Work out the finished part from the listing and answer in its coordinate system (mm). Face numbers are marked on the shaded views. A direction names the side the tool comes from. Round coordinates to 2 decimals unless told otherwise and drop trailing zeros. Loops run counter-clockwise (first coordinate to the right, second up) from the corner with the lowest first, then second, coordinate; pieces in that order, holes last. Notation, with made-up numbers: (23.25, 8.5) -> (56.25, 8.5) arc R26 ccw to (56.25, 43.5) -> close; hole circle Ø6 at (5.25, -21.75). An arc over 180 degrees is marked (long way). Write item = value, one per line. Start each with the question number.
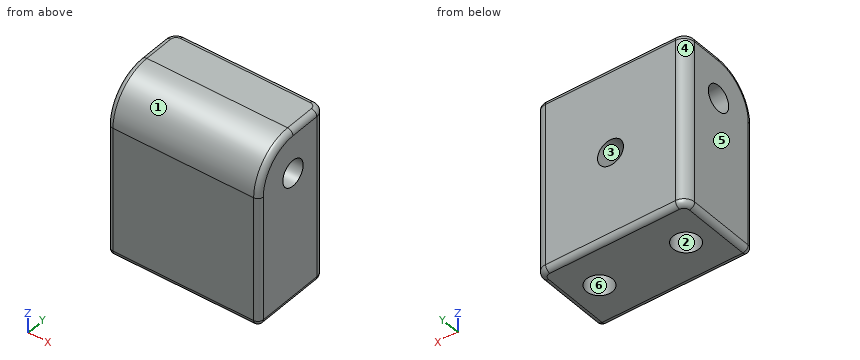
```python
from build123d import *

# Parameters (mm, degrees)
SKETCH1_R           = 1.905
BOSS_EXTRUDE1_DEPTH = 12.7
BOSS_EXTRUDE2_DEPTH = 12.7
CUT_EXTRUDE1_REACH  = 37.955
SKETCH3_R           = 1.905
SKETCH4_R           = 1.905
CUT_EXTRUDE2_DEPTH  = 10.8077
FILLET1_R           = 0.79375
FILLET2_R           = 6.35


with BuildPart() as part:
    # Sketch1 → Boss-Extrude1 (new body)
    with BuildSketch(Plane.XY):
        with BuildLine():
            Line((-11.1125, 0), (11.1125, 0))
            Line((11.1125, 0), (11.1125, 10.8077))
            ThreePointArc((11.1125, 10.8077), (10.647532015, 11.930232015), (9.525, 12.3952))
            Line((9.525, 12.3952), (-9.525, 12.3952))
            ThreePointArc((-9.525, 12.3952), (-10.647532015, 11.930232015), (-11.1125, 10.8077))
            Line((-11.1125, 10.8077), (-11.1125, 0))
        make_face()
        with Locations((-6.35, 6.35)):
            Circle(SKETCH1_R, mode=Mode.SUBTRACT)
        with Locations((6.35, 6.35)):
            Circle(SKETCH1_R, mode=Mode.SUBTRACT)
    extrude(amount=BOSS_EXTRUDE1_DEPTH)

    # Sketch2 → Boss-Extrude2 (add)
    with BuildSketch(Plane.XY.offset(12.7)):
        with BuildLine():
            Line((11.1125, 0), (11.1125, 10.8077))
            ThreePointArc((11.1125, 10.8077), (10.647532015, 11.930232015), (9.525, 12.3952))
            Line((9.525, 12.3952), (-9.525, 12.3952))
            ThreePointArc((-9.525, 12.3952), (-10.647532015, 11.930232015), (-11.1125, 10.8077))
            Line((-11.1125, 10.8077), (-11.1125, 0))
            Line((-11.1125, 0), (11.1125, 0))
        make_face()
    extrude(amount=BOSS_EXTRUDE2_DEPTH)

    # Sketch3 → Cut-Extrude1 (cut, up to next)
    with BuildSketch(Plane(origin=(11.1125, 0, 0), x_dir=(0, 0, -1), z_dir=(1, 0, 0)), mode=Mode.PRIVATE) as cut_extrude1_sk1:
        with Locations(Location((-19.05, 6.35, 0), (0, 0, 90))):
            Circle(SKETCH3_R)
    cut_extrude1_tool1 = extrude(cut_extrude1_sk1.sketch, amount=-CUT_EXTRUDE1_REACH, mode=Mode.PRIVATE) & part.part
    add(cut_extrude1_tool1.solids().sort_by_distance((11.1125, 6.35, 19.05))[0], mode=Mode.SUBTRACT)

    # Sketch4 → Cut-Extrude2 (cut)
    with BuildSketch(Plane(origin=(0, 12.3952, 0), x_dir=(1, 0, 0), z_dir=(0, 1, 0))):
        with Locations(Location((0, -12.7, 0), (0, 0, 180))):
            Circle(SKETCH4_R)
    extrude(amount=-CUT_EXTRUDE2_DEPTH, mode=Mode.SUBTRACT)

    # Fillet1
    fillet1_edges = [part.edges().sort_by_distance(p)[0] for p in [
        (11.1125, 0, 12.7),
        (-11.1125, 0, 12.7),
        (11.1125, 5.40385, 25.4),
        (10.647532015, 11.930232015, 25.4),
        (0, 12.3952, 25.4),
        (-10.647532015, 11.930232015, 25.4),
        (-11.1125, 5.40385, 25.4),
        (0, 0, 0),
        (-11.1125, 5.40385, 0),
        (-10.647532015, 11.930232015, 0),
        (0, 12.3952, 0),
        (10.647532015, 11.930232015, 0),
        (11.1125, 5.40385, 0),
    ]]
    fillet(fillet1_edges, radius=FILLET1_R)

    # Fillet2
    # the kernel refuses this fillet: 6.35 mm, written as the material it takes off along each edge
    with BuildSketch(Plane(origin=(-11.1125, 6.35, 19.05), x_dir=(0, -1, 0), z_dir=(0, 0, -1))) as fillet2_piece_1:
        with BuildLine():
            CenterArc((5.55625, -0.79375), 0.79375, 0, 90)
            Line((6.35, -0.79375), (6.35, 0))
            Line((6.35, 0), (5.55625, 0))
        make_face()
    revolve(axis=Axis((-11.1125, 6.35, 19.05), (-1, 0, 0)), revolution_arc=90, mode=Mode.SUBTRACT)
    with BuildSketch(Plane(origin=(11.1125, 6.35, 19.05), x_dir=(0, 0, 1), z_dir=(0, 1, 0))) as fillet2_piece_2:
        with BuildLine():
            CenterArc((5.55625, -0.79375), 0.79375, 0, 90)
            Line((6.35, -0.79375), (6.35, 0))
            Line((6.35, 0), (5.55625, 0))
        make_face()
    revolve(axis=Axis((11.1125, 6.35, 19.05), (1, 0, 0)), revolution_arc=90, mode=Mode.SUBTRACT)
    with BuildSketch(Plane(origin=(-11.1125, 0, 25.4), x_dir=(0, 0, -1), z_dir=(1, 0, 0))) as fillet2_piece_3:
        with BuildLine():
            CenterArc((FILLET2_R, FILLET2_R), FILLET2_R, 180, 90)
            Line((0, FILLET2_R), (0, 0))
            Line((0, 0), (FILLET2_R, 0))
        make_face()
    extrude(amount=22.225, mode=Mode.SUBTRACT)


solid = part.part
```
Item 1: The mould has two halves that part along Y. Classify the marked faces 1, 2, 3 and 4: pulls with the +Y half, pulls with the -Y half, needs draft (parallel to the pull), parting line crosses it, or undercut.
Item 2: Section D-D (z = 18) is taken. Determine the outline of the cut face in (x, y) (1 decimal), then the cut area to 3 significant figures.
Item 3: Section B-B (z = 10) is taken. Count the separate pieces of the cut face and the enclosed holes in it, then the cut area to 3 significant figures.
Item 4: Find the intervals of material crossed by line 1 along Z through (x, y) = (6.75, 6.35) (3 decimals); line 2 along Z through (x, y) = (0, 5.75) (3 decimals); line 3 along X through (y, z) = (6.75, 11), in increasing order. Write a range as [from, to].
Item 5: A tool of negligible diameter and unlimited length cuts with its end or side. For the marked faces 5 and 6, from which of +Z, -Z, +X, -X, +Y, -Y can it reach the whole face along a straight path? Write none if from no direction.
Item 6: A flat-ended cylindrical pin translates along its axis: pin 1 (1.9 mm diameter, centred on x = -7, y = 6, fed in from -Z). Find the tip coordinate at first contact, or state that the pin passes through.
Worked answers:
q1.face_1 = pulls with the -Y half
q1.face_2 = undercut
q1.face_3 = needs draft
q1.face_4 = pulls with the +Y half
q2.outline = (-11.1, 0.8) arc R0.8 ccw to (-10.3, 0) -> (10.3, 0) arc R0.8 ccw to (11.1, 0.8) -> (11.1, 4.8) -> (-11.1, 4.8) -> close; (-11.1, 7.9) -> (11.1, 7.9) -> (11.1, 10.8) arc R1.6 ccw to (9.5, 12.4) -> (-9.5, 12.4) arc R1.6 ccw to (-11.1, 10.8) -> close
q2.area = 203 mm2
q3.separate_pieces = 1
q3.enclosed_holes = 2
q3.area = 251 mm2
q4.line_1 = [12.7, 17.145], [20.955, 25.4]
q4.line_2 = [0, 10.795], [14.605, 17.242], [20.858, 25.372]
q4.line_3 = [-11.11, -8.21], [-4.49, -0.86], [0.86, 4.49], [8.21, 11.11]
q5.face_5 = +Z, -Z, -X, +Y, -Y
q5.face_6 = -Z
q6.pin_1 = 12.7
